For this review, take the finished solid that the model builds, in its own axes (mm). Face numbers are marked on the shaded views. A direction names the side the tool comes from. Coordinates: 2 decimals unless noted, no trailing zeros. Write each loop counter-clockwise with the first axis right and the second up, starting at its lowest first coordinate (ties: lowest second). Pieces come first, ordered by that corner, then holes. Notation, with made-up numbers: (64, 61.25) - (99, 61.25) arc R27 cw to (99, 83.25) - close; hole circle Ø1 at (-30.75, 83.25). An arc over 180 degrees is marked (long way). Write each question's results on one line, items separated by ' | '.
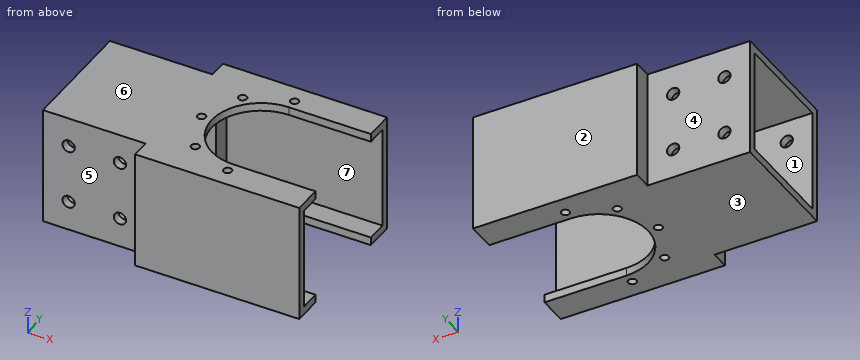
from build123d import *

# Parameters (mm, degrees)
BOSS_EXTRUDE1_DEPTH = 58
SHELL1_T            = -4
SKETCH2_R           = 2
CUT_EXTRUDE1_DEPTH  = 60
SKETCH3_R           = 3
CUT_EXTRUDE2_DEPTH  = 70


with BuildPart() as part:
    # Sketch1 → Boss-Extrude1 (new body)
    with BuildSketch(Plane.XY):
        Polygon((-25, -29), (25, -29), (25, -38), (105, -38), (105, 38), (25, 38), (25, 29), (-25, 29), align=None)
    extrude(amount=BOSS_EXTRUDE1_DEPTH)

    # Shell1
    shell1_openings = [part.faces().sort_by_distance(p)[0] for p in [
        (105, 0, 29),
        (-25, 0, 29),
    ]]
    offset(amount=SHELL1_T, openings=shell1_openings, kind=Kind.INTERSECTION)

    # Sketch2 → Cut-Extrude1 (cut)
    with BuildSketch(Plane(origin=(0, 0, 0), x_dir=(-1, 0, 0), z_dir=(0, 0, -1))):
        with Locations((-36, 0)):
            Circle(SKETCH2_R)
        with Locations((-44.493903346, -20.506096654)):
            Circle(SKETCH2_R)
        with Locations((-65, -29)):
            Circle(SKETCH2_R)
        with Locations((-65, 29)):
            Circle(SKETCH2_R)
        with Locations((-44.493903346, 20.506096654)):
            Circle(SKETCH2_R)
        with BuildLine():
            Line((-65, 24), (-105, 24))
            Line((-105, 24), (-105, -24))
            Line((-105, -24), (-65, -24))
            ThreePointArc((-65, -24), (-41, 0), (-65, 24))
        make_face()
    extrude(amount=-CUT_EXTRUDE1_DEPTH, mode=Mode.SUBTRACT)

    # Sketch3 → Cut-Extrude2 (cut)
    with BuildSketch(Plane.XZ.offset(29)):
        with Locations((12.5, 43.5)):
            Circle(SKETCH3_R)
        with Locations((-12.5, 43.5)):
            Circle(SKETCH3_R)
        with Locations((-12.5, 14.5)):
            Circle(SKETCH3_R)
        with Locations((12.5, 14.5)):
            Circle(SKETCH3_R)
    extrude(amount=-CUT_EXTRUDE2_DEPTH, mode=Mode.SUBTRACT)


solid = part.part
Q1. For the marked faces 4, 5, 6 and 7, list the 3-axis set-ups (+Z, -Z, +X, -X, +Y, -Y) from which the entire face can be reached by the end or side of a thin tool; tool diameter is ignored.
Results found:
face 4: +Z, -Z, -X, +Y | face 5: +Z, -Z, -X, -Y | face 6: +Z, +X, -X, +Y, -Y | face 7: +X
Q2. Take a section at C-C on z = 24. State the section outline as (x, y) points.
Results found:
outline: (-25, -29) - (25, -29) - (25, -38) - (105, -38) - (105, -34) - (29, -34) - (29, -25) - (-25, -25) - close; (-25, 25) - (29, 25) - (29, 34) - (105, 34) - (105, 38) - (25, 38) - (25, 29) - (-25, 29) - close
Q3. Mouldability with a two-part tool opening along Z and no side actions: class the marked faces 1, 2 and 3 as pulls with the +Z half, pulls with the -Z half, needs draft (parallel to the pull), parting line crosses it, or undercut.
Results found:
face 1: undercut | face 2: needs draft | face 3: pulls with the -Z half
Q4. Take a section at B-B on z = 14.5. State how many separate pieces and enclosed holes the cut face has, plus the area to 3 significant figures.
Results found:
separate pieces: 6 | enclosed holes: 0 | area: 1,020 mm2
Q5. Wall thickness on line 1 along Y through (x, z) = (65, 55.7); line 2 along Z through (x, y) = (45, -33.5); line 3 along Y through (x, z) = (-4, 10.5): over which ranges is each line inside the solid? List them lowest first. Write a range as from..to.
Results found:
line 1: -38..-31, -27..-24, 24..27, 31..38 | line 2: 0..4, 54..58 | line 3: -29..-25, 25..29
Q6. For pin 1 (1.5 mm diameter, centred on x = -6, z = 37, fed in from -Y); pin 2 (4.5 mm diameter, centred on y = -31, z = 26.5, fed in from +X); pin 3 (3 mm diameter, centred on y = 22, z = 33, fed in from -X); pin 4 (25 mm diameter, centred on x = 3, z = 18, fed in from +Y), all flat-tipped, find the tip position at first contact; note any pin that passes through.
Results found:
pin 1: y = -29 | pin 2: x = 29 | pin 3: through | pin 4: y = 29
Q7. Take a section at D-D on x = 12.5. State the section outline as (y, z) points, plus the area to 3 significant figures.
Results found:
outline: (-29, 0) - (29, 0) - (29, 11.5) - (25, 11.5) - (25, 4) - (-25, 4) - (-25, 11.5) - (-29, 11.5) - close; (-29, 17.5) - (-25, 17.5) - (-25, 40.5) - (-29, 40.5) - close; (-29, 46.5) - (-25, 46.5) - (-25, 54) - (25, 54) - (25, 46.5) - (29, 46.5) - (29, 58) - (-29, 58) - close; (25, 17.5) - (29, 17.5) - (29, 40.5) - (25, 40.5) - close | area: 768 mm2
Q8. Take a section at A-A on x = 36. State the section outline as (y, z) points, plus the area to 3 significant figures.
Results found:
outline: (-38, 0) - (-2, 0) - (-2, 4) - (-34, 4) - (-34, 54) - (-2, 54) - (-2, 58) - (-38, 58) - close; (2, 0) - (38, 0) - (38, 58) - (2, 58) - (2, 54) - (34, 54) - (34, 4) - (2, 4) - close | area: 976 mm2
